Input: part model. Units: mm. Frame: model coordinates. A direction names the side the tool comes from. Coordinates: 2 decimals unless noted, no trailing zeros. Loops run counter-clockwise (first coordinate to the right, second up) from the corner with the lowest first, then second, coordinate; pieces in that order, holes last.
Item 1: Contact query for a flat-ended pin moving along its axis: P1, Ø1, axis at x = 33, z = 2, coming from the +Y side. Output: stop coordinate, or through.
Item 2: Section C-C on z = 0.55. Return loops of the section in (x, y).
Item 3: Reachability of faces 1 (the cylindrical face through (-13.248, 0.099, 1.479)), 2 (the flat face through (-1, -15, 3)), 3 (the flat face through (-36.9, 48.8, 1.5)), 4 (the flat face through (36.641, 48.574, 1.479)), 5 (the flat face through (-55.995, 23.801, 1.479)) from +Z, -Z, +X, -X, +Y, -Y: full face, straight path, thin tool, end or side. Return the list, or none.
Item 4: Pull-direction query (Y, two-part tool) for faces 6 (the flat face through (56.27, 23.99, 1.48)), 7 (the flat face through (-1, -15, 0)), 8 (the cylindrical face through (-0.29, -8.77, 1.48)), 9 (the cylindrical face through (-3, 0, 1)); classes: released by +Y, released by -Y, zero draft, split by the parting line, or undercut.
Item 5: Ray query, line 1 along Y through (x, z) = (0, 2.2); line 2 along Y through (x, z) = (11, 2.1); line 3 along Y through (x, z) = (-9.5, 0.2). Return the intervals inside material, ascending.
Item 6: Section D-D on x = -57. Return loops of the section in (y, z), and give its area (3 significant figures).
Item 7: Section A-A on y = 0. Return loops of the section in (x, z).
```python
from build123d import *

# Parameters (mm, degrees)
ESQUISSE1_R        = 2.25
ESQUISSE1_R_2      = 3
BOSS_EXTRU_1_DEPTH = 3
CHANFREIN1_SIZE    = 7
CHANFREIN1_SIZE_2  = 6.077264162
CONG_2_R           = 5


with BuildPart() as part:
    # Esquisse1 → Boss.-Extru.1 (new body)
    with BuildSketch(Plane.XY):
        with BuildLine():
            Line((67.003163723, 31.409808199), (52.547583613, 21.418476063))
            ThreePointArc((52.547583613, 21.418476063), (31.520430144, 24.626459013), (33.494666824, 45.805097476))
            Line((33.494666824, 45.805097476), (46.686335037, 57.414163068))
            ThreePointArc((46.686335037, 57.414163068), (0, 74), (-46.686335037, 57.414163068))
            Line((-46.686335037, 57.414163068), (-33.494666824, 45.805097476))
            ThreePointArc((-33.494666824, 45.805097476), (-31.520430144, 24.626459013), (-52.547583613, 21.418476063))
            Line((-52.547583613, 21.418476063), (-67.003163723, 31.409808199))
            ThreePointArc((-67.003163723, 31.409808199), (0, -74), (67.003163723, 31.409808199))
        make_face()
        with Locations((0, 11)):
            Circle(ESQUISSE1_R, mode=Mode.SUBTRACT)
        with Locations((11, 0)):
            Circle(ESQUISSE1_R, mode=Mode.SUBTRACT)
        with Locations((0, -11)):
            Circle(ESQUISSE1_R, mode=Mode.SUBTRACT)
        with Locations((-11, 0)):
            Circle(ESQUISSE1_R, mode=Mode.SUBTRACT)
        Circle(ESQUISSE1_R_2, mode=Mode.SUBTRACT)
    extrude(amount=BOSS_EXTRU_1_DEPTH)

    # Chanfrein1
    # the kernel refuses this chamfer: 7, 6.077264162 mm, written as the material it takes off along each edge
    with BuildSketch(Plane(origin=(-67.003163723, 31.409808199, -18.001780916), x_dir=(0.8226281172410916, -0.5685797927506542, 0), z_dir=(0, 0, 1)), Plane(origin=(46.686335037, 57.414163068, -18.001780916), x_dir=(-0.7507022964494048, -0.660640645211593, 0), z_dir=(0, 0, 1))) as chanfrein1_piece_1:
        with BuildLine():
            Line((CHANFREIN1_SIZE, 0), (1.211839928, -5.788160072))
            ThreePointArc((1.211839928, -5.788160072), (0.563802351, -2.981105416), (0, 0))
            Line((0, 0), (CHANFREIN1_SIZE, 0))
        make_face()
    extrude(amount=39.003561832, mode=Mode.SUBTRACT)
    with BuildSketch(Plane(origin=(-46.686335037, 57.414163068, -17.23797929), x_dir=(0.8036456523944729, 0.5951081123522532, 0), z_dir=(0, 0, 1))) as chanfrein1_piece_2:
        with BuildLine():
            Line((6.703271947, 0), (CHANFREIN1_SIZE_2 * 0.210146029479, -CHANFREIN1_SIZE_2 * 0.977670008946))
            Line((CHANFREIN1_SIZE_2 * 0.210146029479, -CHANFREIN1_SIZE_2 * 0.977670008946), (0, 0))
            ThreePointArc((0, 0), (3.446010548, 0.075880568), (6.703271947, 0))
        make_face()
    extrude(amount=37.475958581, mode=Mode.SUBTRACT)
    with BuildSketch(Plane(origin=(67.003163723, 31.409808199, -17.23797929), x_dir=(-0.8226281172410943, -0.5685797927506503, 0), z_dir=(0, 0, 1))) as chanfrein1_piece_3:
        with BuildLine():
            Line((CHANFREIN1_SIZE_2, 0), (1.408665984, 6.553587944))
            ThreePointArc((1.408665984, 6.553587944), (0.649979278, 3.385007163), (0, 0))
            Line((0, 0), (CHANFREIN1_SIZE_2, 0))
        make_face()
    extrude(amount=37.475958581, mode=Mode.SUBTRACT)

    # Congé2
    cong_2_edges = [part.edges().sort_by_distance(p)[0] for p in [
        (62.003835348, 27.954398601, 1.5),
        (-69.297300979, 25.959277281, 1.5),
        (69.570593152, 25.217703474, 1.5),
        (-41.29927968, 61.403334583, 1.5),
        (41.952710216, 60.958757415, 1.5),
        (41.431418962, 52.789678551, 1.5),
        (-42.124118875, 53.39927535, 1.5),
        (-61.244766903, 27.429749649, 1.5),
    ]]
    fillet(cong_2_edges, radius=CONG_2_R)


solid = part.part
```
Results found:
1. P1: stops at y = 66.48
2. outline: (-70.29, 23.12) arc R74 ccw (long way) to (70.38, 22.87) arc R5 ccw to (67.32, 26.03) - (64.43, 27.08) arc R5 ccw to (59.88, 26.49) - (52.55, 21.42) arc R15.5 cw to (33.49, 45.81) - (39.88, 51.42) arc R5 ccw to (41.56, 54.86) - (41.77, 58.06) arc R5 ccw to (39.44, 62.61) arc R74 ccw to (-39.22, 62.75) arc R5 ccw to (-41.54, 59.02) - (-41.86, 55.96) arc R5 ccw to (-40.19, 51.7) - (-33.49, 45.81) arc R15.5 cw to (-52.55, 21.42) - (-59.54, 26.25) arc R5 ccw to (-63.28, 27.06) - (-66.44, 26.48) arc R5 ccw to start; hole circle Ø4.5 at (-11, 0); hole circle Ø6 at (0, 0); hole circle Ø4.5 at (0, -11); hole circle Ø4.5 at (0, 11); hole circle Ø4.5 at (11, 0)
3. face 1: +Z, -Z
3. face 2: +Z, +X, -X, +Y, -Y
3. face 3: +Z, -Z, -X
3. face 4: +Z, -Z, +X
3. face 5: +Z, -Z, +Y
4. face 6: released by +Y
4. face 7: zero draft
4. face 8: undercut
4. face 9: undercut
5. line 1: y = -74 to -13.25, -8.75 to -3, 3 to 8.75, 13.25 to 74
5. line 2: y = -73.18 to -2.25, 2.25 to 73.18
5. line 3: y = -73.39 to -1.68, 1.68 to 73.39
6. outline: (-47.19, 0) - (24.5, 0) - (24.5, 3) - (-47.19, 3) - close
6. area: 215 mm2
7. outline: (-74, 0) - (-13.25, 0) - (-13.25, 3) - (-74, 3) - close; (-8.75, 0) - (-3, 0) - (-3, 3) - (-8.75, 3) - close; (3, 0) - (8.75, 0) - (8.75, 3) - (3, 3) - close; (13.25, 0) - (74, 0) - (74, 3) - (13.25, 3) - close
